Geometry: final body of the model. Coordinates: model frame, mm. A direction names the side the tool comes from. Round coordinates to 2 decimals unless told otherwise and drop trailing zeros. Loops run counter-clockwise (first coordinate to the right, second up) from the corner with the lowest first, then second, coordinate; pieces in that order, holes last. Notation, with made-up numbers: M -40,38.25 L -14,38.25 A29 ccw -14,75.25 Z; hole C -16,80.25 d1. An arc over 180 degrees is marked long. Answer as a JSON object with one key per item and string values.
```python
from build123d import *

# Parameters (mm, degrees)
SKETCH_1_W          = 25
SKETCH_1_H          = 5
EXTRUDE_1_DEPTH     = 13
SKETCH_2_R          = 12.5
EXTRUDE_2_DEPTH     = 5
CUT_EXTRUDE_1_DEPTH = 5
SKETCH_4_R          = 1.5
CUT_EXTRUDE_2_DEPTH = 5
M3X0_5_1_D          = 2.5
M3X0_5_1_DEPTH      = 10
M3X0_5_1_TIP        = 0.751075774


with BuildPart() as part:
    # ｽｹｯﾁ1 → ﾎﾞｽ - 押し出し1 (new body)
    with BuildSketch(Plane.XY):
        Rectangle(SKETCH_1_W, SKETCH_1_H)
    extrude(amount=EXTRUDE_1_DEPTH)

    # ｽｹｯﾁ2 → ﾎﾞｽ - 押し出し2 (add)
    with BuildSketch(Plane.XZ.offset(2.5)):
        with Locations((0, 13)):
            Circle(SKETCH_2_R)
    extrude(amount=-EXTRUDE_2_DEPTH)

    # ｽｹｯﾁ3 → ｶｯﾄ - 押し出し1 (cut)
    with BuildSketch(Plane(origin=(0, 2.5, 0), x_dir=(1, 0, 0), z_dir=(0, 1, 0))):
        with BuildLine():
            ThreePointArc((-6, -13), (0, -19), (6, -13))
            Line((6, -13), (-6, -13))
        make_face()
        with BuildLine():
            Line((-6, -13), (6, -13))
            ThreePointArc((6, -13), (0, -7), (-6, -13))
        make_face()
    extrude(amount=-CUT_EXTRUDE_1_DEPTH, mode=Mode.SUBTRACT)

    # ｽｹｯﾁ4 → ｶｯﾄ - 押し出し2 (cut)
    with BuildSketch(Plane(origin=(0, 2.5, 0), x_dir=(1, 0, 0), z_dir=(0, 1, 0))):
        with Locations(Location((9, -13, 0), (0, 0, 270))):  # turned: the seam where the file's is
            Circle(SKETCH_4_R)
        with Locations(Location((-9, -13, 0), (0, 0, 270))):  # turned: the seam where the file's is
            Circle(SKETCH_4_R)
    extrude(amount=-CUT_EXTRUDE_2_DEPTH, mode=Mode.SUBTRACT)

    # M3x0.5 ねじ穴1
    with Locations(Plane(origin=(0, 0, 0), x_dir=(-1, 0, 0), z_dir=(0, 0, -1))):
        with Locations((-9, 0), (9, 0)):
            Hole(M3X0_5_1_D / 2, depth=M3X0_5_1_DEPTH)
            with Locations((0, 0, -(M3X0_5_1_DEPTH + M3X0_5_1_TIP / 2))):  # 118° drill point
                Cone(0, M3X0_5_1_D / 2, M3X0_5_1_TIP, mode=Mode.SUBTRACT)


solid = part.part
```
1) Cut plane A-A on z = 9.5. Return the cut outline in (x, y), and give its area (3 significant figures).
Geometry results:
{"outline": "M -12.5,-2.5 L -4.87,-2.5 L -4.87,2.5 L -12.5,2.5 Z; M 4.87,-2.5 L 12.5,-2.5 L 12.5,2.5 L 4.87,2.5 Z; hole C -9,0 d2.5; hole C 9,0 d2.5", "area": "66.4 mm2"}
2) Cut plane C-C on y = 1.75. Return the cut outline in (x, z).
Geometry results:
{"outline": "M -12.5,0 L 12.5,0 L 12.5,13 A12.5 ccw -12.5,13 Z; hole C -9,13 d3; hole C 0,13 d12; hole C 9,13 d3"}
3) Line query: probe 1 along X at (y, z) = (-1.4, 13); probe 2 along X at (y, z) = (1.1, 8.5); probe 3 along Z at (x, y) = (0, -0.1). Output: solid intervals per line, ascending.
Geometry results:
{"probe 1": "-12.5 to -10.5, -7.5 to -6, 6 to 7.5, 10.5 to 12.5", "probe 2": "-12.5 to -9.59, -8.41 to -3.97, 3.97 to 8.41, 9.59 to 12.5", "probe 3": "0 to 7, 19 to 25.5"}
4) First-contact query: pin 1 (1 mm diameter, centred on x = 4, y = -1, fed in from +Z); pin 2 (2 mm diameter, centred on x = 9, y = 0, fed in from +Z). Flat tips, straight axial feed; report the tip coordinate or a pass-through.
Geometry results:
{"pin 1": "z = 25", "pin 2": "z = 22.6"}
5) Set-up query: faces 1 (the face through (-10.25, 0.05, 5.07)), 2 (the face through (12.5, 0, 6)). Return all of +Z, -Z, +X, -X, +Y, -Y with unobstructed straight access to the full face (end or side cutting, diameter ignored); none if empty.
Geometry results:
{"face 1": "-Z", "face 2": "+Z, -Z, +X, +Y, -Y"}
6) Cut plane D-D on z = 2.5. Return the cut outline in (x, y).
Geometry results:
{"outline": "M -12.5,-2.5 L 12.5,-2.5 L 12.5,2.5 L -12.5,2.5 Z; hole C -9,0 d2.5; hole C 9,0 d2.5"}
7) Pull-direction query (X, two-part tool) for faces 3 (the face through (-9.9, 0, 11.8)), 4 (the face through (3, 2.5, 7)), 5 (the face through (8.8, -0.08, 10.62)), 6 (the face through (0.275, -0.035, 25.497)); classes: +X half, -X half, draft (parallel to the pull), parting line (faces both ways), or undercut.
Geometry results:
{"face 3": "undercut", "face 4": "draft", "face 5": "undercut", "face 6": "parting line"}
8) Cut plane B-B on x = 0. Return the cut outline in (y, z).
Geometry results:
{"outline": "M -2.5,0 L 2.5,0 L 2.5,7 L -2.5,7 Z; M -2.5,19 L 2.5,19 L 2.5,25.5 L -2.5,25.5 Z"}
